Input: part model. Units: mm. Frame: model coordinates. A direction names the side the tool comes from. Round coordinates to 2 decimals unless told otherwise and drop trailing zeros. Order: outer loops, then holes, each group sorted by start corner. A loop starts at its lowest first (then second) coordinate and runs counter-clockwise, first axis right, second up. Notation, with made-up numbers: (2.5, 54) -> (54.5, 54) arc R20 ccw to (54.5, 81) -> close; hole circle Ø10 at (-25.5, 23.5). An arc over 180 degrees is marked (long way). Answer as CSV lines item,"result". Start each with the question number.
1) Section query C-C, the plane y = 9. Output: boundary loops of the cut face in (x, z).
2) Mould query, pull axis X, two halves, no side actions, for faces 1 (the face through (11.727, 44.785, -50.521)), 2 (the face through (18, 19, -51)), 3 (the face through (9.13, 4.63, -11.14)). Classes: +X half, -X half, draft (parallel to the pull), parting line (faces both ways), or undercut.
3) First-contact query: P1, Ø4, axis at x = 6, y = 23.5, coming from the +Z side; P2, Ø5, axis at x = 9, z = -67.75, coming from the -Y side; P3, Ø9, axis at x = 10.5, z = -69, coming from the +Y side; P4, Ø8, axis at x = 10.5, y = 36, coming from the -Z side. Flat tips, straight axial feed; report the tip coordinate or a pass-through.
4) Section query A-A, the plane z = -67.75. Output: boundary loops of the cut face in (x, y), and give its area (3 significant figures).
5) Section query D-D, the plane x = 9. Output: boundary loops of the cut face in (y, z), and give its area (3 significant figures).
6) Access query for faces 4 (the face through (6.874, 43.795, -55.108)), 5 (the face through (9.1, 4.1, -70.5)), 6 (the face through (8.874, 21.245, -26.902)). Directions: +Z, -Z, +X, -X, +Y, -Y. A direction counts if a zero-diameter tool reaches every point of the face in a straight line with its end or side. Return the directions, or none.
7) Section query B-B, the plane x = 2. Output: boundary loops of the cut face in (y, z), and give its area (3 significant figures).
8) Line query: L1, parallel to X at y = 4, z = -67.75; L2, parallel to Y at x = 17.25, z = -53.5; L3, parallel to Y at x = 9.5, z = -62. Output: solid intervals per line, ascending.
```python
from build123d import *

# Parameters (mm, degrees)
EXTRUDE_2_DEPTH     = 18
FILLET_2_R          = 1
CUT_EXTRUDE_1_REACH = 93.708
SKETCH_2_R          = 2.75
CUT_EXTRUDE_2_REACH = 97.007
SKETCH_3_R          = 2.75


with BuildPart() as part:
    # 草图1 → 凸台-拉伸2 (new body)
    with BuildSketch(Plane(origin=(0, 0, 0), x_dir=(0, 0, -1), z_dir=(1, 0, 0))):
        Polygon((77, 0), (0, 0), (54.447222151, 54.447222151), (60.104076401, 48.790367902), (47.022600949, 35.70889245), (58.5, 8), (77, 8), align=None)
        Polygon((9.656854249, 4), (56.909677649, 4), (43.069646105, 37.412791856), align=None, mode=Mode.SUBTRACT)
    extrude(amount=EXTRUDE_2_DEPTH)

    # 圆角2
    fillet_2_edges = [part.edges().sort_by_distance(p)[0] for p in [
        (9, 0, 0),
        (9, 37.412791856, -43.069646105),
        (9, 4, -9.656854249),
        (9, 4, -56.909677649),
    ]]
    fillet(fillet_2_edges, radius=FILLET_2_R)

    # 草图2 → 切除-拉伸1 (cut, up to next)
    with BuildSketch(Plane(origin=(0, 8, 0), x_dir=(1, 0, 0), z_dir=(0, 1, 0)), mode=Mode.PRIVATE) as cut_extrude_1_sk1:
        with Locations(Location((9, 67.75, 0), (0, 0, 270))):
            Circle(SKETCH_2_R)
    cut_extrude_1_tool1 = extrude(cut_extrude_1_sk1.sketch, amount=-CUT_EXTRUDE_1_REACH, mode=Mode.PRIVATE) & part.part
    add(cut_extrude_1_tool1.solids().sort_by_distance((9, 8, -67.75))[0], mode=Mode.SUBTRACT)

    # 草图3 → 切除-拉伸2 (cut, up to next)
    with BuildSketch(Plane(origin=(0, -5.656854249, -5.656854249), x_dir=(1, 0, 0), z_dir=(0, -0.7071067811865509, -0.7071067811865441)), mode=Mode.PRIVATE) as cut_extrude_2_sk1:
        with Locations(Location((9, -67.75, 0), (0, 0, 270))):
            Circle(SKETCH_3_R)
    cut_extrude_2_tool1 = extrude(cut_extrude_2_sk1.sketch, amount=-CUT_EXTRUDE_2_REACH, mode=Mode.PRIVATE) & part.part
    add(cut_extrude_2_tool1.solids().sort_by_distance((9, 42.24963, -53.563339))[0], mode=Mode.SUBTRACT)


solid = part.part
```
Findings:
1,outline,"(0, -58.09) -> (18, -58.09) -> (18, -54.84) -> (0, -54.84) -> close; (0, -14.66) -> (18, -14.66) -> (18, -9) -> (0, -9) -> close"
2,face 1,"undercut"
2,face 2,"+X half"
2,face 3,"draft"
3,P1,"stops at z = -21.5"
3,P2,"passes through"
3,P3,"stops at y = 8"
3,P4,"stops at z = -51.31"
4,outline,"(0, 0) -> (6.25, 0) -> (6.25, 8) -> (0, 8) -> close; (11.75, 0) -> (18, 0) -> (18, 8) -> (11.75, 8) -> close"
4,area,"100 mm^2"
5,outline,"(0, -77) -> (8, -77) -> (8, -70.5) -> (0, -70.5) -> close; (0, -65) -> (8, -65) -> (8, -58.5) -> (35.71, -47.02) -> (40.31, -51.62) -> (45.96, -45.96) -> (1.71, -1.71) arc R1 ccw to (0, -2.41) -> close; (44.19, -55.51) -> (48.79, -60.1) -> (54.45, -54.45) -> (49.85, -49.85) -> close; hole (4, -55.41) arc R1 ccw to (5.38, -56.34) -> (36.03, -43.64) arc R1 ccw to (36.35, -42.01) -> (5.71, -11.36) arc R1 ccw to (4, -12.07) -> close"
5,area,"744 mm^2"
6,face 4,"-Z, +X, -X"
6,face 5,"+Y, -Y"
6,face 6,"+X, -X"
7,outline,"(0, -77) -> (8, -77) -> (8, -58.5) -> (35.71, -47.02) -> (48.79, -60.1) -> (54.45, -54.45) -> (1.71, -1.71) arc R1 ccw to (0, -2.41) -> close; hole (4, -55.41) arc R1 ccw to (5.38, -56.34) -> (36.03, -43.64) arc R1 ccw to (36.35, -42.01) -> (5.71, -11.36) arc R1 ccw to (4, -12.07) -> close"
7,area,"832 mm^2"
8,L1,"x = 0 to 6.25, 11.75 to 18"
8,L2,"y = 0 to 4, 12.23 to 20.07, 42.19 to 53.5"
8,L3,"y = 0 to 8"
